from build123d import *

# Parameters (mm, degrees)
BOSS_EXTRUDE1_DEPTH = 20
SKETCH2_R           = 4.2
CUT_EXTRUDE1_DEPTH  = 17.5


with BuildPart() as part:
    # Sketch1 → Boss-Extrude1 (new body)
    with BuildSketch(Plane(origin=(0, 0, 0), x_dir=(0, 1, 0), z_dir=(0, 0, 1))):
        with BuildLine():
            Line((0, 17.937538258), (97.753832512, 8.211917185))
            ThreePointArc((97.753832512, 8.211917185), (105.189280841, 0), (97.753832512, -8.211917185))
            Line((97.753832512, -8.211917185), (0, -17.937538258))
            ThreePointArc((0, -17.937538258), (-19.810719159, 0), (0, 17.937538258))
        make_face()
    extrude(amount=BOSS_EXTRUDE1_DEPTH)

    # Sketch2 → Cut-Extrude1 (cut)
    with BuildSketch(Plane.XY.offset(20)):
        Circle(SKETCH2_R)
    extrude(amount=-CUT_EXTRUDE1_DEPTH, mode=Mode.SUBTRACT)


solid = part.part
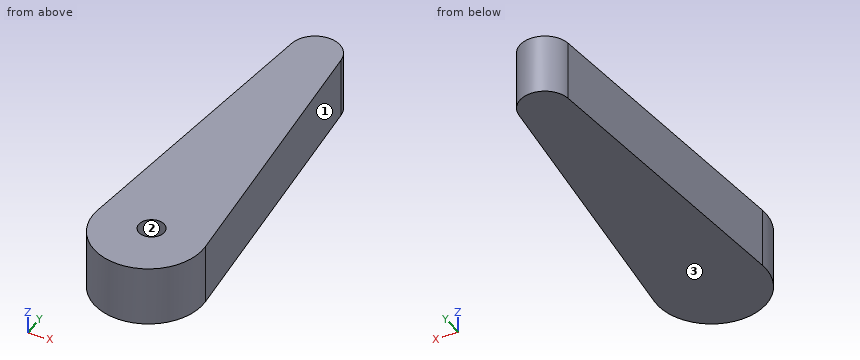
Check sheet for the modelled part. Datum: model origin and axes. Units: mm. Face numbers are marked on the shaded views. Round coordinates to 2 decimals unless told otherwise and drop trailing zeros. Order: outer loops, then holes, each group sorted by start corner. A loop starts at its lowest first (then second) coordinate and runs counter-clockwise, first axis right, second up.
Q1. Depth check by flat-ended pin: P1, Ø6, axis at y = 87.5, z = 17, coming from the -X side; P2, Ø2.5, axis at x = 0, y = 1, coming from the +Z side; P3, Ø4, axis at x = 12, z = 5.5, coming from the -Y side. Enter the tip coordinate at first touch or a pass-through.
Filled sheet:
P1: stops at x = -9.53
P2: stops at z = 2.5
P3: stops at y = -16.78
Q2. Cross-section at D-D, the plane x = 11. Enter the section's corners in (y, z), plus the area to 3 significant figures.
Filled sheet:
outline: (-16.07, 0) - (69.73, 0) - (69.73, 20) - (-16.07, 20) - close
area: 1,720 mm2
Q3. Cross-section at A-A, the plane z = 10.5. Enter the section's corners in (x, y).
Filled sheet:
outline: (-17.94, 0) arc R18.03 ccw (long way) to (17.94, 0) - (8.21, 97.75) arc R8.25 ccw to (-8.21, 97.75) - close; hole circle Ø8.4 at (0, 0)
Q4. Cross-section at C-C, the plane y = 45. Enter the section's corners in (x, z), plus the area to 3 significant figures.
Filled sheet:
outline: (-13.46, 0) - (13.46, 0) - (13.46, 20) - (-13.46, 20) - close
area: 538 mm2
Q5. Draft check along Y on the marked faces 1, 2 and 3. Enter one of: pulls with the +Y half, pulls with the -Y half, needs draft (parallel to the pull), parting line crosses it, or undercut.
Filled sheet:
face 1: pulls with the +Y half
face 2: undercut
face 3: needs draft
Q6. Cross-section at B-B, the plane x = 0. Enter the section's corners in (y, z), plus the area to 3 significant figures.
Filled sheet:
outline: (-19.81, 0) - (105.19, 0) - (105.19, 20) - (4.2, 20) - (4.2, 2.5) - (-4.2, 2.5) - (-4.2, 20) - (-19.81, 20) - close
area: 2,350 mm2
Q7. Scan lines: L1, parallel to X at y = 30, z = 5; L2, parallel to X at y = 94, z = 2.75; L3, parallel to X at y = 0.5, z = 14.5. Record each from-to range of solid material in increasing order.
Filled sheet:
L1: x = -14.95 to 14.95
L2: x = -8.59 to 8.59
L3: x = -17.89 to -4.17, 4.17 to 17.89
